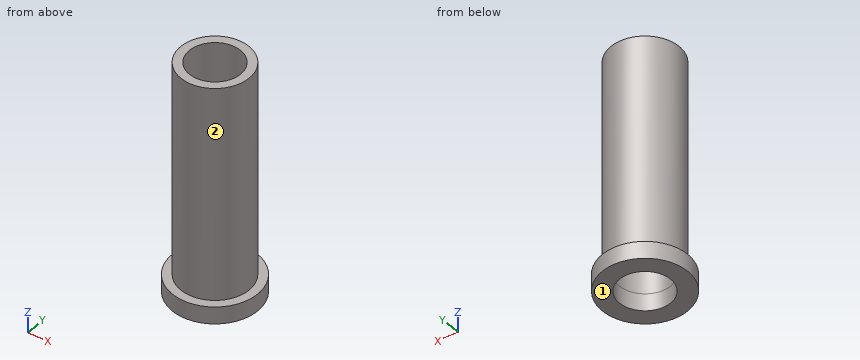
Autodesk Inventor part; units mm, degrees
ref_plane "YZ Plane" through (0, 0, 0) normal (1, 0, 0) x (0, 1, 0)
ref_plane "XZ Plane" through (0, 0, 0) normal (0, 1, 0) x (-1, 0, 0)
ref_plane "XY Plane" through (0, 0, 0) normal (0, 0, 1) x (1, 0, 0)
sketch "Szkic1" plane through (0, 0, 0) normal (0, 0, 1) x (1, 0, 0)
  circle A0 centre (0, 0) radius 3
  circle A1 centre (0, 0) radius 4
  dimension "d0" = 6
  dimension "d1" = 8
extrude "Wyciągnięcie proste1" add sketch "Szkic1" along normal blind 25
sketch "Szkic2" plane through (0, 0, 0) normal (0, 0, -1) x (-1, 0, 0)
  circle A0 centre (0, 0) radius 3
  circle A1 centre (0, 0) radius 5
  dimension "d4" = 6
  dimension "d5" = 10
extrude "Wyciągnięcie proste2" add sketch "Szkic2" along normal blind 2
properties part number "tuleja-palak" material "Mosiądz, miękki żółty"
Read the model definition and answer for the solid it produces. Units are mm, in the model's axes. Face numbers are marked on the shaded views. A direction names the side the tool comes from. Round coordinates to 2 decimals unless told otherwise and drop trailing zeros. Write each loop counter-clockwise with the first axis right and the second up, starting at its lowest first coordinate (ties: lowest second). Pieces come first, ordered by that corner, then holes. Notation, with made-up numbers: (52.25, 65) - (69.25, 65) arc R24 ccw to (69.25, 75) - close; hole circle Ø11 at (31, 26.5). An arc over 180 degrees is marked (long way). One line per question, with ' | ' between items. Start each with the question number.
1. For the marked faces 1 and 2, determine the directions among +Z, -Z, +X, -X, +Y, -Y from which every point of the face is accessible in a straight line to the end or side of a thin tool.
2. Section C-C (z = 16.25) is taken. Determine the outline of the cut face in (x, y).
3. Each of these flat-tipped pins is pushed along its axis until it touches: pin 1 (3 mm diameter, centred on x = -1, z = 15, fed in from +Y); pin 2 (5 mm diameter, centred on y = -0.5, z = 12.5, fed in from +X); pin 3 (2 mm diameter, centred on x = 0.5, z = 17.5, fed in from -Y). Where does it stop, or does it pass through?
4. Section A-A (x = 0) is taken. Determine the outline of the cut face in (y, z).
5. Find the intervals of material crossed by probe 1 along Y at (x, z) = (0, -1.2); probe 2 along Y at (x, z) = (0, 5.75); probe 3 along Z at (x, y) = (-1.5, -3.75), in increasing order. Write a range as [from, to].
Filled in:
1) face 1: -Z, +X, -X, +Y, -Y | face 2: +Z
2) outline: circle Ø8 at (0, 0); hole circle Ø6 at (0, 0)
3) pin 1: y = 4 | pin 2: x = 4 | pin 3: y = -4
4) outline: (-5, -2) - (-3, -2) - (-3, 25) - (-4, 25) - (-4, 0) - (-5, 0) - close; (3, -2) - (5, -2) - (5, 0) - (4, 0) - (4, 25) - (3, 25) - close
5) probe 1: [-5, -3], [3, 5] | probe 2: [-4, -3], [3, 4] | probe 3: [-2, 0]
